Work out the finished part from the listing and answer in its coordinate system (mm). Face numbers are marked on the shaded views. A direction names the side the tool comes from. Round coordinates to 2 decimals unless told otherwise and drop trailing zeros. Loops run counter-clockwise (first coordinate to the right, second up) from the corner with the lowest first, then second, coordinate; pieces in that order, holes last. Notation, with made-up numbers: (38.25, 24.25) - (88.25, 24.25) arc R22 cw to (88.25, 55.25) - close; hole circle Ø3 at (21, -35). An arc over 180 degrees is marked (long way). Return JSON: item names as keys, results as strings.
from build123d import *

# Parameters (mm, degrees)
SKETCH2_R          = 1.016
CUT_EXTRUDE1_DEPTH = 17.655893852
CIRPATTERN1_COUNT  = 2
CIRPATTERN1_ANGLE  = 90


with BuildPart() as part:
    # Sketch1 → Revolve1 (revolve)
    with BuildSketch(Plane(origin=(0, 0, 0), x_dir=(1, 0, 0), z_dir=(0, 1, 0)), mode=Mode.PRIVATE) as revolve1_sk:
        Polygon((-10.16, 3.3655), (0, 3.3655), (2.309689752, 2.032), (12.7, 2.032), (12.7, 5.08), (3.81, 5.08), (0, 7.62), (-10.16, 7.62), align=None)
    revolve(revolve1_sk.sketch.rotate(Axis((0, 0, 0), (1, 0, 0)), 180), axis=Axis((0, 0, 0), (1, 0, 0)))

    # Sketch2 → Cut-Extrude1 (cut, through all)
    with BuildSketch(Plane(origin=(0, 0, 0), x_dir=(1, 0, 0), z_dir=(0, 1, 0))):
        with Locations(Location((-5.08, 0, 0), (0, 0, 90))):
            Circle(SKETCH2_R)
        with Locations(Location((8.255, 0, 0), (0, 0, 90))):
            Circle(SKETCH2_R)
    cut_extrude1 = extrude(amount=CUT_EXTRUDE1_DEPTH, mode=Mode.SUBTRACT)

    # CirPattern1: Cut-Extrude1 ×2 about axis
    cirpattern1_axis = Axis((-10.16, 0, 0), (-1, 0, 0))
    for i in range(1, CIRPATTERN1_COUNT):
        add(cut_extrude1.rotate(cirpattern1_axis, i * CIRPATTERN1_ANGLE / (CIRPATTERN1_COUNT - 1)), mode=Mode.SUBTRACT)


solid = part.part
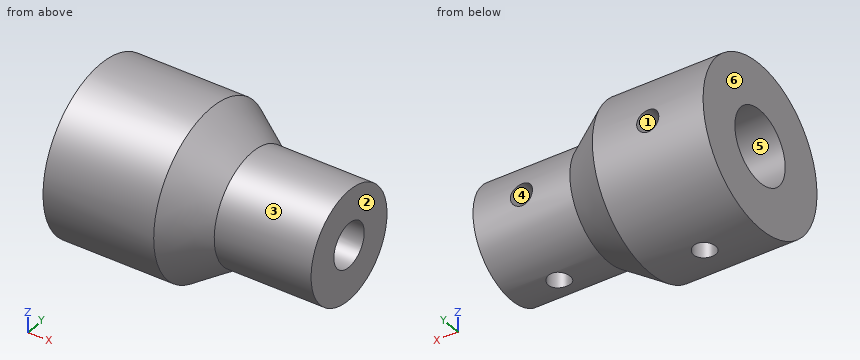
1) Determine the mould class of the marked faces 1, 2 and 3 for opening direction Z: pulls with the +Z half, pulls with the -Z half, needs draft (parallel to the pull), parting line crosses it, or undercut.
Verdict:
{"face 1": "undercut", "face 2": "needs draft", "face 3": "parting line crosses it"}
2) Section A-A (z = 0) is taken. Give the vertices of the cut face in (x, y), and give its area (3 significant figures).
Verdict:
{"outline": "(-10.16, -7.62) - (0, -7.62) - (3.81, -5.08) - (12.7, -5.08) - (12.7, -2.03) - (2.31, -2.03) - (0, -3.37) - (-10.16, -3.37) - close; (-10.16, 3.37) - (-6.1, 3.37) - (-6.1, 7.62) - (-10.16, 7.62) - close; (-4.06, 3.37) - (0, 3.37) - (2.31, 2.03) - (7.24, 2.03) - (7.24, 5.08) - (3.81, 5.08) - (0, 7.62) - (-4.06, 7.62) - close; (9.27, 2.03) - (12.7, 2.03) - (12.7, 5.08) - (9.27, 5.08) - close", "area": "156 mm2"}
3) Flat-ended cylindrical pins translate along their axes: pin 1 (3.5 mm diameter, centred on y = 0, z = 0, fed in from +X); pin 2 (1.6 mm diameter, centred on x = 8.255, y = 0, fed in from -Z); pin 3 (1.5 mm diameter, centred on x = 10, y = 4, fed in from +Z); pin 4 (5 mm diameter, centred on x = 1, y = -4, fed in from -Z). Find the tip coordinate at first contact, or state that the pin passes through.
Verdict:
{"pin 1": "passes through", "pin 2": "stops at z = 1.87", "pin 3": "stops at z = 3.9", "pin 4": "stops at z = -7.43"}
4) Section D-D (x = 3.5) is taken. Give the vertices of the cut face in (y, z).
Verdict:
{"outline": "circle Ø10.57 at (0, 0); hole circle Ø4.06 at (0, 0)"}
5) Find the intervals of material crossed by L1, parallel to X at y = 0, z = -4.55; L2, parallel to Y at x = -3.75, z = 0; L3, parallel to Y at x = 4, z = -1, in increasing order.
Verdict:
{"L1": "x = -10.16 to -6.1, -4.06 to 7.24, 9.27 to 12.7", "L2": "y = -7.62 to -3.37, 3.37 to 7.62", "L3": "y = -4.98 to -1.77, 1.77 to 4.98"}
6) Section B-B (x = -5.08) is taken. Give the vertices of the cut face in (y, z).
Verdict:
{"outline": "(-1.02, -7.55) - (-1.02, -3.21) arc R3.37 cw (long way) to (3.21, 1.02) - (7.55, 1.02) arc R7.62 ccw (long way) to start; (1.02, -7.55) arc R7.62 ccw to (7.55, -1.02) - (3.21, -1.02) arc R3.37 cw to (1.02, -3.21) - close"}
7) A tool of negligible diameter and unlimited length cuts with its end or side. For the marked faces 4, 5 and 6, from which of +Z, -Z, +X, -X, +Y, -Y can it reach the whole face along a straight path? Write none if from no direction.
Verdict:
{"face 4": "+Y", "face 5": "-X", "face 6": "+Z, -Z, -X, +Y, -Y"}
8) Section C-C (x = 0.5) is taken. Give the vertices of the cut face in (y, z), and give its area (3 significant figures).
Verdict:
{"outline": "circle Ø14.57 at (0, 0); hole circle Ø6.15 at (0, 0)", "area": "137 mm2"}
